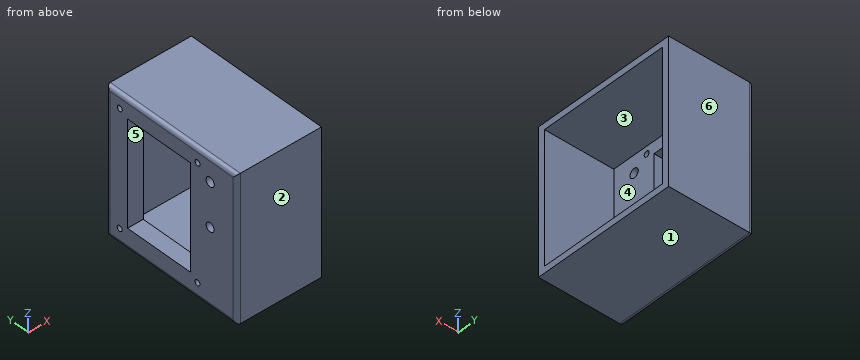
from build123d import *

# Parameters (mm, degrees)
ESBO_O1_W                = 100
ESBO_O1_H                = 100
ESBO_O1_R                = 2.099999731
ESBO_O1_R_2              = 3.499999496
ESBO_O1_R_3              = 3.399999765
RESSALTO_EXTRUS_O1_DEPTH = 12
ESBO_O2_W                = 80
ESBO_O2_H                = 53
CORTE_EXTRUS_O1_DEPTH    = 12
ESBO_O3_W                = 110
ESBO_O3_H                = 110
ESBO_O3_W_2              = 100
ESBO_O3_H_2              = 100
RESSALTO_EXTRUS_O2_DEPTH = 65
FILETE1_R                = 3


with BuildPart() as part:
    # Esboço1 → Ressalto-extrusão1 (new body)
    with BuildSketch(Plane(origin=(0, 0, 0), x_dir=(0, 0, -1), z_dir=(1, 0, 0))):
        with Locations((-414.454548573, 389.240771296)):
            Rectangle(ESBO_O1_W, ESBO_O1_H)
        with Locations((-371.077987612, 432.946200958)):
            Circle(ESBO_O1_R, mode=Mode.SUBTRACT)
        with Locations((-371.024063379, 367.14624515)):
            Circle(ESBO_O1_R, mode=Mode.SUBTRACT)
        with Locations((-458.877958129, 432.87424738)):
            Circle(ESBO_O1_R, mode=Mode.SUBTRACT)
        with Locations((-458.824033895, 367.074291572)):
            Circle(ESBO_O1_R, mode=Mode.SUBTRACT)
        with Locations((-451.165348634, 356.487124133)):
            Circle(ESBO_O1_R_2, mode=Mode.SUBTRACT)
        with Locations((-418.165360481, 356.508431567)):
            Circle(ESBO_O1_R_3, mode=Mode.SUBTRACT)
    extrude(amount=RESSALTO_EXTRUS_O1_DEPTH)

    # Esboço2 → Corte-extrusão1 (cut)
    with BuildSketch(Plane.ZY):
        with Locations((415.220911045, 399.798918519)):
            Rectangle(ESBO_O2_W, ESBO_O2_H)
    extrude(amount=-CORTE_EXTRUS_O1_DEPTH, mode=Mode.SUBTRACT)

    # Esboço3 → Ressalto-extrusão2 (add)
    with BuildSketch(Plane.ZY):
        with Locations((414.454548573, 389.240771296)):
            Rectangle(ESBO_O3_W, ESBO_O3_H)
        with Locations((414.454548573, 389.240771296)):
            Rectangle(ESBO_O3_W_2, ESBO_O3_H_2, mode=Mode.SUBTRACT)
    extrude(amount=-RESSALTO_EXTRUS_O2_DEPTH)

    # Filete1
    filete1_edges = [part.edges().sort_by_distance(p)[0] for p in [
        (0, 444.240771296, 414.454548573),
        (0, 389.240771296, 359.454548573),
        (0, 334.240771296, 414.454548573),
        (0, 389.240771296, 469.454548573),
    ]]
    fillet(filete1_edges, radius=FILETE1_R)


solid = part.part
Build history of the part. All positions in model axes, mm. Face numbers are marked on the shaded views. A direction names the side the tool comes from. Give positions to 0.01 mm unless a question says otherwise; leave off trailing zeros. Order: outer loops, then holes, each group sorted by start corner. A loop starts at its lowest first (then second) coordinate and runs counter-clockwise, first axis right, second up. Notation, with made-up numbers: M 77.5,20 L 97.5,20 A18 cw 97.5,36 Z; hole C 38.25,64 d7. An arc over 180 degrees is marked long. Use one line per item in the form item = value.
1) Saw through at D-D (y = 344.5). Give the cut face in (x, z), plus the area to 3 significant figures.
Calculated:
outline = M 0,362.45 A3 ccw 3,359.45 L 65,359.45 L 65,364.45 L 12,364.45 L 12,464.45 L 65,464.45 L 65,469.45 L 3,469.45 A3 ccw 0,466.45 Z
area = 1,850 mm2
2) Tool access for the marked faces 4, 5 and 6: list every direction of +Z, -Z, +X, -X, +Y, -Y with a clear straight run to the whole face (end or side of a thin tool).
Calculated:
face_4 = +X
face_5 = +X, -X
face_6 = +Z, -Z, +X, -X, +Y
3) Saw through at C-C (x = 47). Give the cut face in (y, z), plus the area to 3 significant figures.
Calculated:
outline = M 334.24,359.45 L 444.24,359.45 L 444.24,469.45 L 334.24,469.45 Z; hole M 339.24,364.45 L 439.24,364.45 L 439.24,464.45 L 339.24,464.45 Z
area = 2,100 mm2
4) Probe probe 1 along Z at (x, y) = (47.5, 398); probe 2 along Y at (x, z) = (24, 422.5); probe 3 along Y at (x, z) = (9, 390.5). List the from-to ranges inside material, lowest first.
Calculated:
probe_1 = 359.45 to 364.45, 464.45 to 469.45
probe_2 = 334.24 to 339.24, 439.24 to 444.24
probe_3 = 334.24 to 373.3, 426.3 to 444.24
5) Saw through at B-B (y = 376). Give the cut face in (x, z).
Calculated:
outline = M 0,362.45 A3 ccw 3,359.45 L 65,359.45 L 65,364.45 L 12,364.45 L 12,375.22 L 0,375.22 Z; M 0,455.22 L 12,455.22 L 12,464.45 L 65,464.45 L 65,469.45 L 3,469.45 A3 ccw 0,466.45 Z
6) Drop flat-ended pins along their axis: pin 1 (6 mm diameter, centred on y = 431.5, z = 450, fed in from +X); pin 2 (4 mm diameter, centred on y = 432.95, z = 371.08, fed in from +X); pin 3 (5 mm diameter, centred on y = 367.15, z = 371.02, fed in from -X). Give the stop position or say it passes through.
Calculated:
pin_1 = 12
pin_2 = through
pin_3 = 0
7) Two-plate mould, pull along Y, no slides. Class the marked faces 1, 2 and 3: released by +Y, released by -Y, zero draft, split by the parting line, or undercut.
Calculated:
face_1 = zero draft
face_2 = released by -Y
face_3 = undercut
8) Saw through at A-A (z = 389). Give the cut face in (x, y).
Calculated:
outline = M 0,337.24 A3 ccw 3,334.24 L 65,334.24 L 65,339.24 L 12,339.24 L 12,373.3 L 0,373.3 Z; M 0,426.3 L 12,426.3 L 12,439.24 L 65,439.24 L 65,444.24 L 3,444.24 A3 ccw 0,441.24 Z
